Source: CAD feature listing. Evaluate the final solid. Frame: model axes, mm. Face numbers are marked on the shaded views. A direction names the side the tool comes from. Round coordinates to 2 decimals unless told otherwise and drop trailing zeros. Loops run counter-clockwise (first coordinate to the right, second up) from the corner with the lowest first, then second, coordinate; pieces in that order, holes last. Notation, with made-up numbers: M -3.5,50.25 L 2.5,50.25 A10 cw 2.5,68.25 Z; hole C -20,88.25 d3. An arc over 180 degrees is marked long. Answer as a JSON object with one key per item and string values.
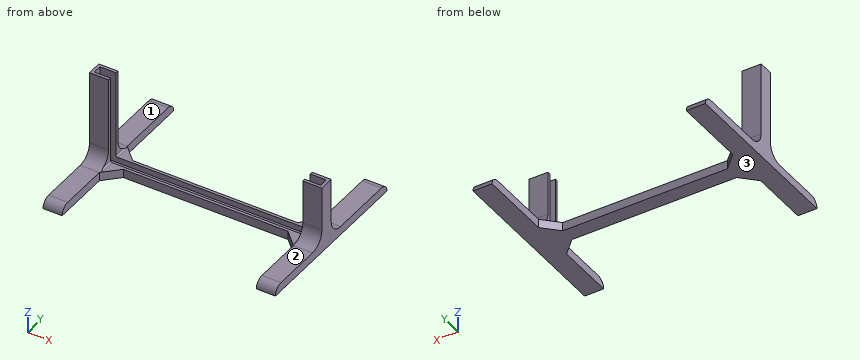
from build123d import *

# Parameters (mm, degrees)
F0_W         = 200.66
F0_H         = 3.7321411073
F1_DEPTH     = 12.7
F2_T         = -2.54
F3_W         = 16.51
F3_H         = 7.4579973676
F4_DEPTH     = 76.2
F6_START     = 11.176
F5_W         = 16.51
F5_H         = 7.4579973676
F6_DEPTH     = 65.024
F7_T1_DEPTH  = 7.4579973676
F8_T1_DEPTH  = 16.51
F8_T3_DEPTH  = 16.51
F9_T1_DEPTH  = 2.54
F9_T3_DEPTH  = 2.54
F9_T8_DEPTH  = 22.225
F9_S9_R      = 12.6999999999
F9_T10_DEPTH = 13
F9_T15_DEPTH = 22.225
F9_S16_R     = 12.6999999999
F9_T17_DEPTH = 13
F9_T22_DEPTH = 22.225
F9_S24_R     = 12.6999999999
F9_T25_DEPTH = 13
F9_T29_DEPTH = 22.225
F9_S31_R     = 12.6999999999
F9_T32_DEPTH = 13
F10_T1_DEPTH = 54.6013885108
F10_T3_DEPTH = 54.6013885108


# Not quite as in the source:
# - a fillet or chamfer that OpenCascade refuses, or shapes differently, is made with other operations: its cross-section is extruded or revolved along the edge and cut away or added


with BuildPart() as f1:
    # F0 (on Front) → F1 (new body)
    with BuildSketch(Plane.XZ):
        Polygon((83.82, -55.5934350035), (-83.82, -55.5934350035), (-83.82, 20.6065649965), (-100.33, 20.6065649965), (-100.33, -59.3192912638), (100.33, -59.3192912638), (100.33, -4.7934350035), (83.82, -4.7934350035), align=None)
        with Locations((0, -61.1853618175)):
            Rectangle(F0_W, F0_H)
    extrude(amount=F1_DEPTH)

    # F2
    f2_openings = [f1.faces().sort_by_distance(p)[0] for p in [
        (-92.075, -6.35, 20.606565),
        (-83.82, -6.35, -17.493435),
        (0, -6.35, -55.593435),
        (92.075, -6.35, -4.793435),
        (83.82, -6.35, -30.193435),
    ]]
    offset(amount=F2_T, openings=f2_openings)

    # F3 (on Front) → F4 (join)
    with BuildSketch(Plane.XZ):
        with Locations((92.075, -59.3224336873)):
            Rectangle(F3_W, F3_H)
        with Locations((-92.075, -59.3224336873)):
            Rectangle(F3_W, F3_H)
    extrude(amount=-F4_DEPTH)

    # F5 (on Front) → F6 (join)
    with BuildSketch(Plane.XZ.offset(F6_START)):
        with Locations((-92.075, -59.3224336873)):
            Rectangle(F5_W, F5_H)
        with Locations((92.075, -59.3224336873)):
            Rectangle(F5_W, F5_H)
    extrude(amount=F6_DEPTH)

    # F7: chamfer of 12.7 on 4 edges, made by hand

    # F7_s2 → F7_t1 (join)
    with BuildSketch(Plane.XY.offset(-63.0514323711)):
        Polygon((-71.12, -12.7), (-83.82, -25.4), (-83.82, -12.7), align=None)
        Polygon((-83.82, 12.7), (-71.12, 0), (-83.82, 0), align=None)
        Polygon((71.12, 0), (83.82, 12.7), (83.82, 0), align=None)
        Polygon((71.12, -12.7), (83.82, -25.4), (83.82, -12.7), align=None)
    extrude(amount=F7_T1_DEPTH)

    # F8: fillet of radius 12.7 on 4 edges, made by hand

    # F8_s2 → F8_t1 (join)
    with BuildSketch(Plane.YZ.offset(-100.33)):
        with BuildLine():
            ThreePointArc((-12.7, -42.8934350035), (-16.4197438789, -51.8736911246), (-25.4, -55.5934350035))
            Line((-25.4, -55.5934350035), (-12.7, -55.5934350035))
            Line((-12.7, -55.5934350035), (-12.7, -42.8934350035))
        make_face()
        with BuildLine():
            ThreePointArc((0, -42.8934350035), (3.7197438789, -51.8736911246), (12.7, -55.5934350035))
            Line((12.7, -55.5934350035), (0, -55.5934350035))
            Line((0, -55.5934350035), (0, -42.8934350035))
        make_face()
    extrude(amount=F8_T1_DEPTH)

    # F8_s4 → F8_t3 (join)
    with BuildSketch(Plane.YZ.offset(83.82)):
        with BuildLine():
            ThreePointArc((-25.4, -55.5934350035), (-16.4197438789, -51.8736911246), (-12.7, -42.8934350035))
            Line((-12.7, -42.8934350035), (-12.7, -55.5934350035))
            Line((-12.7, -55.5934350035), (-25.4, -55.5934350035))
        make_face()
        with BuildLine():
            ThreePointArc((12.7, -55.5934350035), (3.7197438789, -51.8736911246), (0, -42.8934350035))
            Line((0, -42.8934350035), (0, -55.5934350035))
            Line((0, -55.5934350035), (12.7, -55.5934350035))
        make_face()
    extrude(amount=F8_T3_DEPTH)

    # F9: fillet of radius 1.27 on 8 edges, made by hand

    # F9_s2 → F9_t1 (join)
    with BuildSketch(Plane.XZ):
        with BuildLine():
            ThreePointArc((-83.82, -54.3234350035), (-83.4480256121, -55.2214606156), (-82.55, -55.5934350035))
            Line((-82.55, -55.5934350035), (-83.82, -55.5934350035))
            Line((-83.82, -55.5934350035), (-83.82, -54.3234350035))
        make_face()
        with BuildLine():
            ThreePointArc((82.55, -55.5934350035), (83.4480256121, -55.2214606156), (83.82, -54.3234350035))
            Line((83.82, -54.3234350035), (83.82, -55.5934350035))
            Line((83.82, -55.5934350035), (82.55, -55.5934350035))
        make_face()
    extrude(amount=F9_T1_DEPTH)

    # F9_s4 → F9_t3 (join)
    with BuildSketch(Plane.XZ.offset(10.16)):
        with BuildLine():
            ThreePointArc((-83.82, -54.3234350035), (-83.4480256121, -55.2214606156), (-82.55, -55.5934350035))
            Line((-82.55, -55.5934350035), (-83.82, -55.5934350035))
            Line((-83.82, -55.5934350035), (-83.82, -54.3234350035))
        make_face()
        with BuildLine():
            ThreePointArc((82.55, -55.5934350035), (83.4480256121, -55.2214606156), (83.82, -54.3234350035))
            Line((83.82, -54.3234350035), (83.82, -55.5934350035))
            Line((83.82, -55.5934350035), (82.55, -55.5934350035))
        make_face()
    extrude(amount=F9_T3_DEPTH)


with BuildPart() as f9_tool6:
    # F9_s7 → F9_t8 (new body)
    with BuildSketch(Plane.XZ.offset(-22.225)):
        with BuildLine():
            ThreePointArc((-83.82, -54.3234350035), (-83.4480256121, -55.2214606156), (-82.55, -55.5934350035))
            Line((-82.55, -55.5934350035), (-83.82, -55.5934350035))
            Line((-83.82, -55.5934350035), (-83.82, -54.3234350035))
        make_face()
    extrude(amount=F9_T8_DEPTH)

    # F9_s9 → F9_t10 (cut, symmetric)
    with BuildSketch(Plane.YZ.offset(-83.2)):
        with Locations((12.6999999999, -42.8934350036)):
            Circle(F9_S9_R)
    extrude(amount=F9_T10_DEPTH, both=True, mode=Mode.SUBTRACT)

    split(bisect_by=Plane(origin=(-35.56, -35.56, 0), x_dir=(0, 0, 1), z_dir=(-0.7071067812, -0.7071067812, 0)), keep=Keep.TOP)


with BuildPart() as f1_1:
    add(f1.part)

    # F9_t5: union F9_tool6
    add(f9_tool6.part)


with BuildPart() as f9_tool13:
    # F9_s14 → F9_t15 (new body)
    with BuildSketch(Plane.XZ.offset(34.925)):
        with BuildLine():
            ThreePointArc((-83.82, -54.3234350035), (-83.4480256121, -55.2214606156), (-82.55, -55.5934350035))
            Line((-82.55, -55.5934350035), (-83.82, -55.5934350035))
            Line((-83.82, -55.5934350035), (-83.82, -54.3234350035))
        make_face()
    extrude(amount=-F9_T15_DEPTH)

    # F9_s16 → F9_t17 (cut, symmetric)
    with BuildSketch(Plane.YZ.offset(-83.2)):
        with Locations((-25.3999999999, -42.8934350036)):
            Circle(F9_S16_R)
    extrude(amount=F9_T17_DEPTH, both=True, mode=Mode.SUBTRACT)

    split(bisect_by=Plane(origin=(-29.21, 29.21, 0), x_dir=(0, 0, 1), z_dir=(-0.7071067812, 0.7071067812, 0)), keep=Keep.TOP)


with BuildPart() as f1_2:
    add(f1_1.part)

    # F9_t12: union F9_tool13
    add(f9_tool13.part)


with BuildPart() as f9_tool20:
    # F9_s21 → F9_t22 (new body)
    with BuildSketch(Plane.XZ):
        with BuildLine():
            ThreePointArc((82.55, -55.5934350035), (83.4480256121, -55.2214606156), (83.82, -54.3234350035))
            Line((83.82, -54.3234350035), (83.82, -55.5934350035))
            Line((83.82, -55.5934350035), (82.55, -55.5934350035))
        make_face()
    extrude(amount=-F9_T22_DEPTH)

    split(bisect_by=Plane(origin=(35.56, -35.56, 0), x_dir=(0, 0, 1), z_dir=(0.7071067812, -0.7071067812, 0)), keep=Keep.TOP)

    # F9_s24 → F9_t25 (cut, symmetric)
    with BuildSketch(Plane.YZ.offset(83.2)):
        with Locations((12.6999999999, -42.8934350036)):
            Circle(F9_S24_R)
    extrude(amount=F9_T25_DEPTH, both=True, mode=Mode.SUBTRACT)


with BuildPart() as f1_3:
    add(f1_2.part)

    # F9_t19: union F9_tool20
    add(f9_tool20.part)


with BuildPart() as f9_tool27:
    # F9_s28 → F9_t29 (new body)
    with BuildSketch(Plane.XZ.offset(12.7)):
        with BuildLine():
            ThreePointArc((82.55, -55.5934350035), (83.4480256121, -55.2214606156), (83.82, -54.3234350035))
            Line((83.82, -54.3234350035), (83.82, -55.5934350035))
            Line((83.82, -55.5934350035), (82.55, -55.5934350035))
        make_face()
    extrude(amount=F9_T29_DEPTH)

    split(bisect_by=Plane(origin=(29.21, 29.21, 0), x_dir=(0, 0, 1), z_dir=(0.7071067812, 0.7071067812, 0)), keep=Keep.TOP)

    # F9_s31 → F9_t32 (cut, symmetric)
    with BuildSketch(Plane.YZ.offset(83.2)):
        with Locations((-25.3999999999, -42.8934350036)):
            Circle(F9_S31_R)
    extrude(amount=F9_T32_DEPTH, both=True, mode=Mode.SUBTRACT)


with BuildPart() as f1_4:
    add(f1_3.part)

    # F9_t26: union F9_tool27
    add(f9_tool27.part)

    # F10: fillet of radius 7.62 on 4 edges, made by hand

    # F10_s2 → F10_t1 (cut)
    with BuildSketch(Plane.YZ.offset(-119.3756942554)):
        with BuildLine():
            ThreePointArc((68.5817222978, -55.5934350035), (73.9122916831, -57.7683059849), (76.2, -63.0514323711))
            Line((76.2, -63.0514323711), (76.2, -55.5934350035))
            Line((76.2, -55.5934350035), (68.5817222978, -55.5934350035))
        make_face()
        with BuildLine():
            ThreePointArc((-76.2, -63.0514323711), (-73.9122916831, -57.7683059849), (-68.5817222978, -55.5934350035))
            Line((-68.5817222978, -55.5934350035), (-76.2, -55.5934350035))
            Line((-76.2, -55.5934350035), (-76.2, -63.0514323711))
        make_face()
    extrude(amount=F10_T1_DEPTH, mode=Mode.SUBTRACT)

    # F10_s4 → F10_t3 (cut)
    with BuildSketch(Plane.YZ.offset(64.7743057446)):
        with BuildLine():
            ThreePointArc((68.5817222978, -55.5934350035), (73.9122916831, -57.7683059849), (76.2, -63.0514323711))
            Line((76.2, -63.0514323711), (76.2, -55.5934350035))
            Line((76.2, -55.5934350035), (68.5817222978, -55.5934350035))
        make_face()
        with BuildLine():
            ThreePointArc((-68.5817222978, -55.5934350035), (-73.9122916831, -57.7683059849), (-76.2, -63.0514323711))
            Line((-76.2, -63.0514323711), (-76.2, -55.5934350035))
            Line((-76.2, -55.5934350035), (-68.5817222978, -55.5934350035))
        make_face()
    extrude(amount=F10_T3_DEPTH, mode=Mode.SUBTRACT)


solid = f1_4.part
Item 1: Line query: probe 1 along Y at (x, z) = (-90.5, -14); probe 2 along Z at (x, y) = (85.5, -2); probe 3 along Y at (x, z) = (81.5, -57). Output: solid intervals per line, ascending. Write a range as from..to.
Answer sheet:
{"probe 1": "y = -12.7..-10.16, -2.54..0", "probe 2": "z = -63.05..-4.79", "probe 3": "y = -23.08..-10.16, -2.54..10.38"}
Item 2: Section D-D on z = 7. Return the cut outline in (x, y), then the cut area to 3 significant figures.
Answer sheet:
{"outline": "M -100.33,-12.7 L -83.82,-12.7 L -83.82,-10.16 L -97.79,-10.16 L -97.79,-2.54 L -83.82,-2.54 L -83.82,0 L -100.33,0 Z", "area": "103 mm²"}
Item 3: Section A-A on z = -28. Return the cut outline in (x, y).
Answer sheet:
{"outline": "M -100.33,-12.7 L -83.82,-12.7 L -83.82,-10.16 L -97.79,-10.16 L -97.79,-2.54 L -83.82,-2.54 L -83.82,0 L -100.33,0 Z; M 83.82,-12.7 L 100.33,-12.7 L 100.33,0 L 83.82,0 L 83.82,-2.54 L 97.79,-2.54 L 97.79,-10.16 L 83.82,-10.16 Z"}
Item 4: Contact query for flat-ended pins moving along their axis: pin 1 Ø13 at (x, z) = (-94, -22.5) entering from -Y; pin 2 Ø5 at (x, z) = (-92.5, -23) entering from +Y; pin 3 Ø8 at (y, z) = (-28.5, -49) entering from +X; pin 4 Ø6.5 at (x, y) = (95, -3.5) entering from +Z. Output: stop coordinate, or through.
Answer sheet:
{"pin 1": "stops at y = -12.7", "pin 2": "stops at y = 0", "pin 3": "passes through", "pin 4": "stops at z = -4.79"}
Item 5: Access query for the marked faces 1, 2 and 3. Directions: +Z, -Z, +X, -X, +Y, -Y. A direction counts if a zero-diameter tool reaches every point of the face in a straight line with its end or side. Return the directions, or none.
Answer sheet:
{"face 1": "+Z, +X, -X, +Y", "face 2": "+Z, +X, -X, -Y", "face 3": "-Z, +X, -X, +Y, -Y"}
Item 6: Section B-B on y = -32.5. Return the cut outline in (x, z), then the cut area to 3 significant figures.
Answer sheet:
{"outline": "M -100.33,-63.05 L -83.82,-63.05 L -83.82,-55.59 L -100.33,-55.59 Z; M 83.82,-63.05 L 100.33,-63.05 L 100.33,-55.59 L 83.82,-55.59 Z", "area": "246 mm²"}
Item 7: Section C-C on x = 75. Return the cut outline in (y, z), then the cut area to 3 significant figures.
Answer sheet:
{"outline": "M -16.58,-63.05 L 3.88,-63.05 L 3.88,-55.59 L -2.54,-55.59 L -2.54,-60.51 L -10.16,-60.51 L -10.16,-55.59 L -16.58,-55.59 Z", "area": "115 mm²"}
